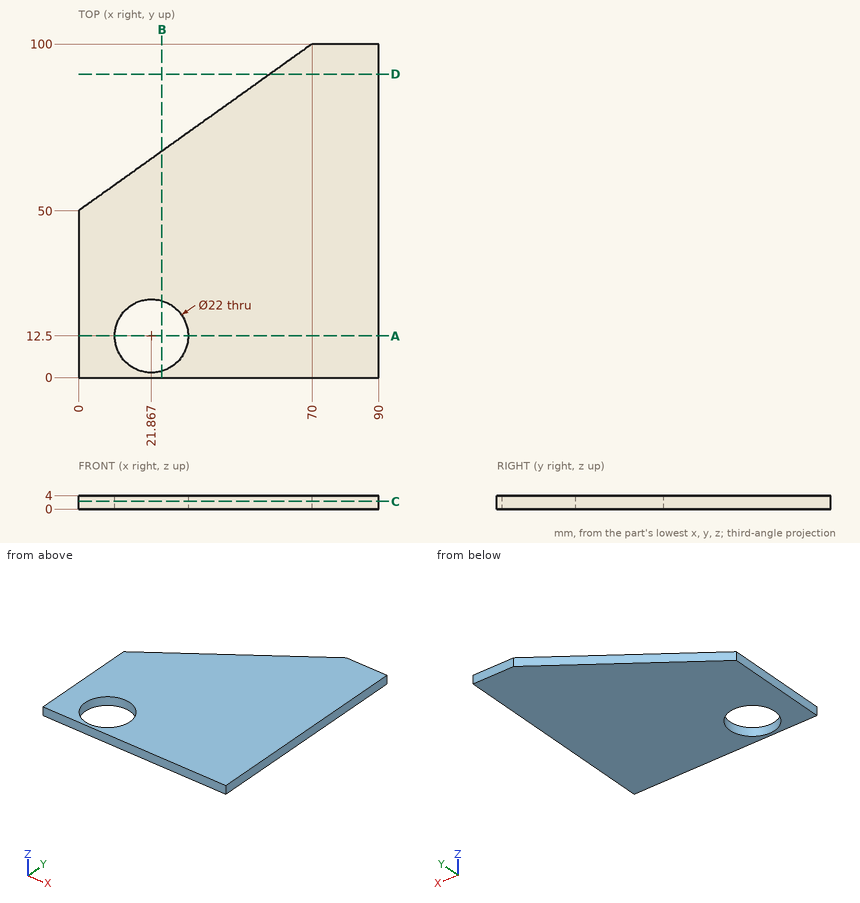
Check sheet for the drawn part. Datum: minimum x, y, z corner. Units: mm. Give positions to 0.01 mm unless a question says otherwise; leave off trailing zeros. Order: outer loops, then holes, each group sorted by start corner. A loop starts at its lowest first (then second) coordinate and runs counter-clockwise, first axis right, second up. Notation, with made-up numbers: (-18.5, 23) - (-13.5, 23) arc R18 ccw to (-13.5, 30) - close; hole circle Ø1 at (49.5, -34.5). An arc over 180 degrees is marked (long way). Answer as a JSON object with one key per item and string values.
(1) Cross-section at D-D (y = 91). Record the cut outline in (x, z), then the cut area to 3 significant figures.
Report:
{"outline": "(57.4, 0) - (90, 0) - (90, 4) - (57.4, 4) - close", "area": "130 mm^2"}
(2) Cross-section at A-A (y = 12.5). Record the cut outline in (x, z), then the cut area to 3 significant figures.
Report:
{"outline": "(0, 0) - (10.87, 0) - (10.87, 4) - (0, 4) - close; (32.87, 0) - (90, 0) - (90, 4) - (32.87, 4) - close", "area": "272 mm^2"}
(3) Cross-section at B-B (x = 25). Record the cut outline in (y, z).
Report:
{"outline": "(0, 0) - (1.96, 0) - (1.96, 4) - (0, 4) - close; (23.04, 0) - (67.86, 0) - (67.86, 4) - (23.04, 4) - close"}
(4) Material ranges on line 1 (Y direction, x = 56, z = 0.45); line 2 (Y direction, x = 30, z = 2.35); line 3 (Y direction, x = 14, z = 2.55), recorded low to high.
Report:
{"line 1": "0 to 90", "line 2": "0 to 5.09, 19.91 to 71.43", "line 3": "0 to 4.81, 20.19 to 60"}
(5) Depth check by flat-ended pin: pin 1 Ø20 at (x, y) = (21.87, 12.5) entering from +Z. Enter the tip coordinate at first touch or a pass-through.
Report:
{"pin 1": "through"}
(6) Cross-section at C-C (z = 2.3). Record the cut outline in (x, y), then the cut area to 3 significant figures.
Report:
{"outline": "(0, 0) - (90, 0) - (90, 100) - (70, 100) - (0, 50) - close; hole circle Ø22 at (21.87, 12.5)", "area": "6,870 mm^2"}
